Verification items for the finished model (mm, model axes). A direction names the side the tool comes from. Round coordinates to 2 decimals unless told otherwise and drop trailing zeros. Order: outer loops, then holes, each group sorted by start corner. A loop starts at its lowest first (then second) coordinate and runs counter-clockwise, first axis right, second up. Notation, with made-up numbers: (37, -33) -> (60, -33) arc R15 ccw to (60, -19) -> close; hole circle Ø8 at (42.25, 2). An arc over 180 degrees is marked (long way). Put each result on its own line as item: value.
```python
from build123d import *

# Parameters (mm, degrees)
SKETCH1_R       = 7.2771
EXTRUDE3_DEPTH  = 3.81
SKETCH4_W       = 19.05
SKETCH4_H       = 3.175
CHAMFER2_SIZE   = 0.9525
SKETCH26_R      = 0.5461
EXTRUDE13_DEPTH = 3.794184746


with BuildPart() as part:
    # Sketch1 → Extrude3 (new body)
    with BuildSketch(Plane.XY):
        with Locations(Location((0, 0, 0), (0, 0, 180))):
            Circle(SKETCH1_R)
    extrude(amount=EXTRUDE3_DEPTH)

    # Sketch11 → Cut-Revolve3 (revolve, cut)
    with BuildSketch(Plane(origin=(0, 0, 0), x_dir=(0, 0, -1), z_dir=(1, 0, 0)), mode=Mode.PRIVATE) as cut_revolve3_sk:
        with BuildLine():
            Line((-4.064, 8.73252), (0, 8.73252))
            Line((0, 8.73252), (0, 7.2771))
            Line((0, 7.2771), (-0.381, 7.2771))
            ThreePointArc((-0.381, 7.2771), (-2.909812836, 4.022257619), (-3.81, 0))
            Line((-3.81, 0), (-4.064, 0))
            Line((-4.064, 0), (-4.064, 8.73252))
        make_face()
    revolve(cut_revolve3_sk.sketch.rotate(Axis((0, 0, 0), (0, 0, 1)), 90), axis=Axis((0, 0, 0), (0, 0, 1)), mode=Mode.SUBTRACT)



with BuildPart() as body_2:
    # Sketch4 → Revolve1 (revolve)
    with BuildSketch(Plane(origin=(0, 0, 0), x_dir=(0, 0, -1), z_dir=(1, 0, 0))):
        with Locations((9.525, 1.5875)):
            Rectangle(SKETCH4_W, SKETCH4_H)
    revolve(axis=Axis((0, 0, 0), (0, 0, -1)))

    # Chamfer2
    chamfer2_edges = [body_2.edges().sort_by_distance(p)[0] for p in [
        (0, -3.175, -19.05),
    ]]
    chamfer(chamfer2_edges, length=CHAMFER2_SIZE)


with BuildPart() as part_1:
    add(part.part)

    add(body_2.part)  # Extrude13 merges body 2
    # Sketch26 → Extrude13 (add)
    with BuildSketch(Plane.XY):
        Circle(SKETCH26_R)
    extrude(amount=EXTRUDE13_DEPTH)


solid = part_1.part
```
Item 1: Sectioned sample at D-D, the plane y = 6.5. Record the boundary of the cut face in (x, z).
Geometry check:
outline: (-3.27, 0) -> (3.27, 0) -> (3.27, 0.38) arc R6.84 ccw to (-3.27, 0.38) -> close
Item 2: Tool access check on faces 1 (the face through (-3, 2, 0)), 2 (the face through (-6.94, -2.19, 0.19)). Record the directions out of +Z, -Z, +X, -X, +Y, -Y that give a thin tool (end or side, any length) a straight path to the whole face; none if there is none.
Geometry check:
face 1: -Z
face 2: +Z, -Z
Item 3: Depth check by flat-ended pin: pin 1 Ø5 at (y, z) = (-4.5, -13.5) entering from -X; pin 2 Ø2 at (x, z) = (-2, -3) entering from +Y; pin 3 Ø5 at (y, z) = (-0.5, -15.5) entering from +X (3 decimals). Enter the tip coordinate at first touch or a pass-through.
Geometry check:
pin 1: x = -2.47
pin 2: y = 3.01
pin 3: x = 3.175
Item 4: Material ranges on line 1 along Z through (x, y) = (6, -3.25); line 2 along X through (y, z) = (-1.5, -5.5); line 3 along Z through (x, y) = (-6, 0.5), recorded low to high.
Geometry check:
line 1: 0 to 0.89
line 2: -2.8 to 2.8
line 3: 0 to 1.64
Item 5: Sectioned sample at C-C, the plane z = -9.5. Record the boundary of the cut face in (x, y) (3 decimals).
Geometry check:
outline: circle Ø6.35 at (0, 0)
